from build123d import *

# Parameters (mm, degrees)
SKETCH1_R           = 3.375
BOSS_EXTRUDE1_DEPTH = 1.65
SKETCH2_R           = 1.5
BOSS_EXTRUDE2_DEPTH = 6.35
CHAMFER1_SIZE       = 0.3
CUT_EXTRUDE1_DEPTH  = 2
CHAMFER2_SIZE       = 1.65


with BuildPart() as part:
    # Sketch1 → Boss-Extrude1 (new body)
    with BuildSketch(Plane.XY):
        Circle(SKETCH1_R)
    extrude(amount=BOSS_EXTRUDE1_DEPTH)

    # Sketch2 → Boss-Extrude2 (add)
    with BuildSketch(Plane(origin=(0, 0, 0), x_dir=(-1, 0, 0), z_dir=(0, 0, -1))):
        with Locations(Location((0, 0, 0), (0, 0, 180))):
            Circle(SKETCH2_R)
    extrude(amount=BOSS_EXTRUDE2_DEPTH)

    # Chamfer1
    chamfer1_edges = [part.edges().sort_by_distance(p)[0] for p in [
        (-1.5, 0, -6.35),
    ]]
    chamfer(chamfer1_edges, length=CHAMFER1_SIZE)

    # Sketch3 → Cut-Extrude1 (cut)
    with BuildSketch(Plane.XY.offset(1.65)):
        Polygon((0, 1.154700538), (-1, 0.577350269), (-1, -0.577350269), (0, -1.154700538), (1, -0.577350269), (1, 0.577350269), align=None)
    extrude(amount=-CUT_EXTRUDE1_DEPTH, mode=Mode.SUBTRACT)

    # Chamfer2
    chamfer2_edges = [part.edges().sort_by_distance(p)[0] for p in [
        (-3.375, 0, 0),
    ]]
    chamfer(chamfer2_edges, length=CHAMFER2_SIZE - 0.0001)  # a hair under: the kernel refuses the full size


solid = part.part
Input: part model. Units: mm. Frame: model coordinates. A direction names the side the tool comes from. Give positions to 0.01 mm unless a question says otherwise; leave off trailing zeros. Order: outer loops, then holes, each group sorted by start corner. A loop starts at its lowest first (then second) coordinate and runs counter-clockwise, first axis right, second up. Notation, with made-up numbers: (36.5, 21.25) - (49.5, 21.25) arc R15 cw to (49.5, 28.25) - close; hole circle Ø5 at (85, -0.75). An arc over 180 degrees is marked (long way). Answer as a JSON object with one key per item and string values. Group by question number.
Q1. Mould query, pull axis X, two halves, no side actions, for faces 3 (the face through (1, 1, 1.65)), 4 (the face through (1.43, -0.45, -2.98)), 5 (the face through (0.51, 0.86, 0.66)). Classes: pulls with the +X half, pulls with the -X half, needs draft (parallel to the pull), parting line crosses it, or undercut.
Q2. Set-up query: faces 1 (the face through (0, 0, -6.35)), 2 (the face through (-0.51, -0.86, 0.66)). Return all of +Z, -Z, +X, -X, +Y, -Y with unobstructed straight access to the full face (end or side cutting, diameter ignored); none if empty.
Q3. First-contact query: pin 1 Ø3 at (y, z) = (2, -3.5) entering from +X; pin 2 Ø3 at (x, z) = (2, -3) entering from -Y; pin 3 Ø1 at (y, z) = (-1, -2) entering from -X. Flat tips, straight axial feed; report the tip coordinate or a pass-through.
Q4. Cut plane B-B, the plane z = -3.25. Output: boundary loops of the cut face in (x, y).
Q5. Line query: probe 1 along Y at (x, z) = (0, -3.75); probe 2 along X at (y, z) = (-0.75, 1.25); probe 3 along Z at (x, y) = (0.25, -0.25). Output: solid intervals per line, ascending.
Results:
{
 "1": {"face 3": "needs draft", "face 4": "parting line crosses it", "face 5": "undercut"},
 "2": {"face 1": "-Z, +X, -X, +Y, -Y", "face 2": "+Z"},
 "3": {"pin 1": "x = 1.41", "pin 2": "y = -1.41", "pin 3": "x = -1.41"},
 "4": {"outline": "circle Ø3 at (0, 0)"},
 "5": {"probe 1": "-1.5 to 1.5", "probe 2": "-2.88 to -0.7, 0.7 to 2.88", "probe 3": "-6.35 to -0.35"}
}
